Geometry: final body of the model. Coordinates: model frame, mm. Coordinates: 2 decimals unless noted, no trailing zeros. Order: outer loops, then holes, each group sorted by start corner. A loop starts at its lowest first (then second) coordinate and runs counter-clockwise, first axis right, second up. Notation, with made-up numbers: M 23.5,65 L 66.5,65 A30 ccw 66.5,96 Z; hole C 58.5,30 d3. An arc over 180 degrees is marked long. Use CSV: the item, a comma, the result in double quotes. Start each with the question number.
1. Material intervals for line 1 (X direction, y = -12, z = 212); line 2 (Z direction, x = 507, y = -9.75); line 3 (X direction, y = -14, z = 279), sorted ascending.
2. Pull-direction query (X, two-part tool) for faces 1 (the flat face through (294, -6, 0)), 2 (the flat face through (76, -9, 297)), 3 (the flat face through (0, -6, 294)), 4 (the flat face through (596, -6, 294)); classes: pulls with the +X half, pulls with the -X half, needs draft (parallel to the pull), parting line crosses it, or undercut.
3. Section query A-A on x = 441. Return the cut outline in (y, z), and give its area (3 significant figures).
4. Section query B-B on z = 264. Return the cut outline in (x, y), and give its area (3 significant figures).
from build123d import *

# Parameters (mm, degrees)
F0_W      = 44.656470418
F0_H      = 33.8078811765
F1_DEPTH  = 16
F2_DEPTH  = 796
F3_DEPTH  = 196
F4_W      = 68.9578056335
F4_H      = 493.6993122101
F5_DEPTH  = 7
F6_DEPTH  = 9.7
F7_DEPTH  = 99.33
F8_DEPTH  = 99.33
F9_DEPTH  = 17.34
F10_DEPTH = 102.97
F11_W     = 35.2807044983
F11_H     = 492.0964837074
F12_DEPTH = 7
F13_DEPTH = 37.27
F14_DEPTH = 6.58
F15_DEPTH = 106.63
F16_DEPTH = 5.87
F17_DEPTH = 200
F18_DEPTH = 200
F19_DEPTH = 200
F20_DEPTH = 200
F21_DEPTH = 200
F22_DEPTH = 200
F23_DEPTH = 200
F24_DEPTH = 200
F25_DEPTH = 200
F26_R     = 3


with BuildPart() as f1:
    # F0 (on Front) → F1 (new body)
    with BuildSketch(Plane.XZ):
        with Locations((22.328235209, 16.9039405882)):
            Rectangle(F0_W, F0_H)
    extrude(amount=F1_DEPTH)

    # F2 (add): a face of the model
    f2_faces = [f1.faces().sort_by_distance(p)[0] for p in [
        (22.328235209, -8, 0),
    ]]
    extrude(f2_faces, amount=-F2_DEPTH)

    # F3 (add): a face of the model
    f3_faces = [f1.faces().sort_by_distance(p)[0] for p in [
        (0, -8, 398),
    ]]
    extrude(f3_faces, amount=-F3_DEPTH)

    # F4 (on face) → F5 (cut)
    with BuildSketch(Plane.XZ.offset(16)):
        with Locations((94.1769480705, 399.8196721077)):
            Rectangle(F4_W, F4_H)
    extrude(amount=-F5_DEPTH, mode=Mode.SUBTRACT)

    # F6 (cut): a face of the model
    f6_faces = [f1.faces().sort_by_distance(p)[0] for p in [
        (59.6980452538, -12.5, 399.8196721077),
    ]]
    extrude(f6_faces, amount=-F6_DEPTH, mode=Mode.SUBTRACT)

    # F7 (add): a face of the model
    f7_faces = [f1.faces().sort_by_distance(p)[0] for p in [
        (89.3269480705, -12.5, 646.6693282127),
    ]]
    extrude(f7_faces, amount=-F7_DEPTH)

    # F8 (cut): a face of the model
    f8_faces = [f1.faces().sort_by_distance(p)[0] for p in [
        (89.3269480705, -12.5, 646.6693282127),
    ]]
    extrude(f8_faces, amount=-F8_DEPTH, mode=Mode.SUBTRACT)

    # F9 (cut): a face of the model
    f9_faces = [f1.faces().sort_by_distance(p)[0] for p in [
        (128.6558508873, -12.5, 449.4846721077),
    ]]
    extrude(f9_faces, amount=-F9_DEPTH, mode=Mode.SUBTRACT)

    # F10 (cut): a face of the model
    f10_faces = [f1.faces().sort_by_distance(p)[0] for p in [
        (97.9969480705, -12.5, 152.9700160027),
    ]]
    extrude(f10_faces, amount=-F10_DEPTH, mode=Mode.SUBTRACT)

    # F11 (on face) → F12 (join)
    with BuildSketch(Plane.XZ.offset(9)):
        with Locations((91.7714834213, 432.6795041561)):
            Rectangle(F11_W, F11_H)
    extrude(amount=F12_DEPTH)

    # F13 (add): a face of the model
    f13_faces = [f1.faces().sort_by_distance(p)[0] for p in [
        (91.7714834213, -12.5, 678.7277460098),
    ]]
    extrude(f13_faces, amount=F13_DEPTH)

    # F14 (add): a face of the model
    f14_faces = [f1.faces().sort_by_distance(p)[0] for p in [
        (109.4118356705, -12.5, 451.3145041561),
    ]]
    extrude(f14_faces, amount=F14_DEPTH)

    # F15 (add): a face of the model
    f15_faces = [f1.faces().sort_by_distance(p)[0] for p in [
        (95.0614834213, -12.5, 186.6312623024),
    ]]
    extrude(f15_faces, amount=F15_DEPTH)

    # F16 (cut): a face of the model
    f16_faces = [f1.faces().sort_by_distance(p)[0] for p in [
        (74.1311311722, -12.5, 397.9995041561),
    ]]
    extrude(f16_faces, amount=-F16_DEPTH, mode=Mode.SUBTRACT)

    # F17 (add): a face of the model
    f17_faces = [f1.faces().sort_by_distance(p)[0] for p in [
        (196, -8, 398),
    ]]
    extrude(f17_faces, amount=F17_DEPTH)

    # F18 (cut): a face of the model
    f18_faces = [f1.faces().sort_by_distance(p)[0] for p in [
        (145.9958508873, -12.5, 397.9996721077),
    ]]
    extrude(f18_faces, amount=-F18_DEPTH, mode=Mode.SUBTRACT)

    # F19 (add): a face of the model
    f19_faces = [f1.faces().sort_by_distance(p)[0] for p in [
        (115.9918356705, -12.5, 397.9995041561),
    ]]
    extrude(f19_faces, amount=F19_DEPTH)

    # F20 (add): a face of the model
    f20_faces = [f1.faces().sort_by_distance(p)[0] for p in [
        (396, -8, 398),
    ]]
    extrude(f20_faces, amount=F20_DEPTH)

    # F21 (cut): a face of the model
    f21_faces = [f1.faces().sort_by_distance(p)[0] for p in [
        (345.9958508873, -12.5, 397.9996721077),
    ]]
    extrude(f21_faces, amount=-F21_DEPTH, mode=Mode.SUBTRACT)

    # F22 (add): a face of the model
    f22_faces = [f1.faces().sort_by_distance(p)[0] for p in [
        (315.9918356705, -12.5, 397.9995041561),
    ]]
    extrude(f22_faces, amount=F22_DEPTH)

    # F23 (cut): a face of the model
    f23_faces = [f1.faces().sort_by_distance(p)[0] for p in [
        (297.9964834213, -12.5, 715.9977460098),
    ]]
    extrude(f23_faces, amount=-F23_DEPTH, mode=Mode.SUBTRACT)

    # F24 (add): a face of the model
    f24_faces = [f1.faces().sort_by_distance(p)[0] for p in [
        (297.9969480705, -12.5, 745.9993282127),
    ]]
    extrude(f24_faces, amount=F24_DEPTH)

    # F25 (cut): a face of the model
    f25_faces = [f1.faces().sort_by_distance(p)[0] for p in [
        (298, -8, 796),
    ]]
    extrude(f25_faces, amount=-F25_DEPTH, mode=Mode.SUBTRACT)

    # F26
    f26_edges = [f1.edges().sort_by_distance(p)[0] for p in [
        (0, -16, 298),
        (298, -16, 596),
        (596, -16, 298),
        (298, -16, 0),
        (49.998045, -16, 297.999672),
        (297.996948, -16, 50.000016),
        (297.996948, -16, 545.999328),
        (545.995851, -16, 297.999672),
        (297.996483, -16, 515.997746),
        (515.991836, -16, 297.999504),
        (297.996483, -16, 80.001262),
        (80.001131, -16, 297.999504),
    ]]
    fillet(f26_edges, radius=F26_R)


solid = f1.part
Results list:
1,line 1,"x = 0 to 50, 80 to 515.99, 546 to 596"
1,line 2,"z = 0 to 50, 80 to 516, 546 to 596"
1,line 3,"x = 0.17 to 49.83, 80.17 to 515.82, 546.17 to 595.83"
2,face 1,"needs draft"
2,face 2,"undercut"
2,face 3,"pulls with the -X half"
2,face 4,"pulls with the +X half"
3,outline,"M -16,3 A3 ccw -13,0 L 0,0 L 0,596 L -13,596 A3 ccw -16,593 L -16,549 A3 ccw -13,546 L -9,546 L -9,516 L -13,516 A3 ccw -16,513 L -16,83 A3 ccw -13,80 L -9,80 L -9,50 L -13,50 A3 ccw -16,47 Z"
3,area,"9,100 mm²"
4,outline,"M 0,-13 A3 ccw 3,-16 L 47,-16 A3 ccw 50,-13 L 50,-9 L 80,-9 L 80,-13 A3 ccw 83,-16 L 512.99,-16 A3 ccw 515.99,-13 L 515.99,-9 L 546,-9 L 546,-13 A3 ccw 549,-16 L 593,-16 A3 ccw 596,-13 L 596,0 L 0,0 Z"
4,area,"9,100 mm²"
